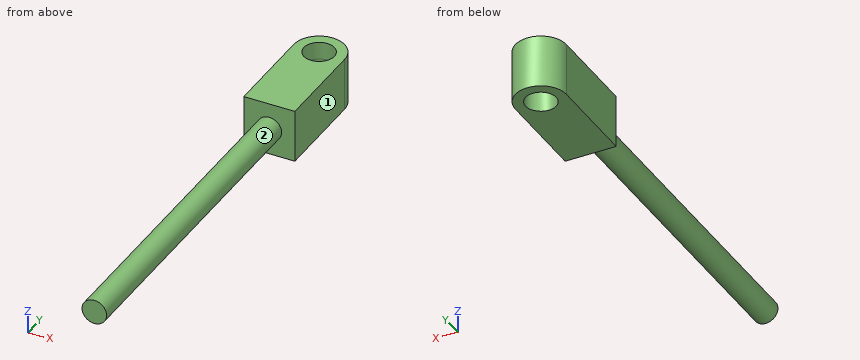
from build123d import *

# Parameters (mm, degrees)
SKETCH1_R                = 1.5
BOSS_EXTRUDE1_DEPTH      = 1.725
BOSS_EXTRUDE1_DEPTH_BACK = 3.45
SKETCH2_R                = 1.203
BOSS_EXTRUDE2_DEPTH      = 32.5


with BuildPart() as part:
    # Sketch1 → Boss-Extrude1 (new body, two sides)
    with BuildSketch(Plane.XY) as boss_extrude1_sk:
        with BuildLine():
            Line((-2.5, 0), (-2.5, -9.25))
            Line((-2.5, -9.25), (2.5, -9.25))
            Line((2.5, -9.25), (2.5, 0))
            ThreePointArc((2.5, 0), (0, 2.5), (-2.5, 0))
        make_face()
        Circle(SKETCH1_R, mode=Mode.SUBTRACT)
    extrude(amount=BOSS_EXTRUDE1_DEPTH)
    extrude(boss_extrude1_sk.sketch, amount=-BOSS_EXTRUDE1_DEPTH_BACK)

    # Sketch2 → Boss-Extrude2 (add)
    with BuildSketch(Plane.XZ.offset(9.25)):
        with Locations((0, -0.8625)):
            Circle(SKETCH2_R)
    extrude(amount=BOSS_EXTRUDE2_DEPTH)


solid = part.part
Source: CAD feature listing. Evaluate the final solid. Frame: model axes, mm. Face numbers are marked on the shaded views. A direction names the side the tool comes from. Coordinates: 2 decimals unless noted, no trailing zeros. Loops run counter-clockwise (first coordinate to the right, second up) from the corner with the lowest first, then second, coordinate; pieces in that order, holes last. Notation, with made-up numbers: (70, 30.5) -> (78, 30.5) arc R13 cw to (78, 53.5) -> close; hole circle Ø5 at (7.5, 32.25). An arc over 180 degrees is marked (long way). Answer in a Markdown table with one row per item. Add a question column.
Q1. Section B-B on z = 0.9. Return the cut outline in (x, y), and give its area (3 significant figures).
Q2. Reachability of the marked faces 1 and 2 from +Z, -Z, +X, -X, +Y, -Y: full face, straight path, thin tool, end or side. Return the list, or none.
Q3. Ray query, line 1 along Y through (x, z) = (0, -1.5); line 2 along Y through (x, z) = (0, 1.3); line 3 along Y through (x, z) = (2, -2.05). Return the intervals inside material, ascending.
Q4. Section D-D on y = -38. Return the cut outline in (x, z), and give its area (3 significant figures).
Q5. Contact query for flat-ended pins moving along their axis: pin 1 Ø2 at (y, z) = (-36.5, -2.5) entering from +X; pin 2 Ø2.5 at (x, y) = (0, 0) entering from +Z; pin 3 Ø3 at (y, z) = (-16.5, 0.5) entering from -X. Output: stop coordinate, or through.
Q6. Section C-C on z = -1.7. Return the cut outline in (x, y).
Computed values:
| question | item | result |
|---|---|---|
| 1 | outline | (-2.5, -9.25) -> (2.5, -9.25) -> (2.5, 0) arc R2.5 ccw to (-2.5, 0) -> close; hole circle Ø3 at (0, 0) |
| 1 | area | 49.0 mm^2 |
| 2 | face 1 | +Z, -Z, +X, +Y, -Y |
| 2 | face 2 | -Y |
| 3 | line 1 | y = -41.75 to -1.5, 1.5 to 2.5 |
| 3 | line 2 | y = -9.25 to -1.5, 1.5 to 2.5 |
| 3 | line 3 | y = -9.25 to 1.5 |
| 4 | outline | circle Ø2.41 at (0, -0.86) |
| 4 | area | 4.55 mm^2 |
| 5 | pin 1 | stops at x = 1.02 |
| 5 | pin 2 | passes through |
| 5 | pin 3 | stops at x = -1.2 |
| 6 | outline | (-2.5, -9.25) -> (-0.86, -9.25) -> (-0.86, -41.75) -> (0.86, -41.75) -> (0.86, -9.25) -> (2.5, -9.25) -> (2.5, 0) arc R2.5 ccw to (-2.5, 0) -> close; hole circle Ø3 at (0, 0) |
